Autodesk Fusion 360 part; units mm, degrees
sketch "Sketch1" plane through (0, 0, 0) normal (0, 0, 1) x (1, 0, 0)
  circle A0 centre (0, 0) radius 45.72 construction
  circle A1 centre (22.86, 39.5947) radius 4.4196
  line L0 (0, 0) -> (0, 63.5) construction
  line L1 (22.86, 39.5947) -> (0, 0) construction
  line L2 (0, 0) -> (69.088, 0) construction
  circle A2 centre (-22.86, 39.5947) radius 4.4196
  circle A3 centre (-45.72, 0) radius 4.4196
  circle A4 centre (-22.86, -39.5947) radius 4.4196
  circle A5 centre (22.86, -39.5947) radius 4.4196
  arc A6 (-14.8961, 45.9035) -> (-32.3056, 35.8522) centre (-22.86, 39.5947) ccw
  arc A7 (-47.2017, 10.0514) -> (-47.2017, -10.0514) centre (-45.72, 0) ccw
  arc A8 (-32.3056, -35.8522) -> (-14.8961, -45.9035) centre (-22.86, -39.5947) ccw
  line L3 (55.88, 55.88) -> (55.88, -43.18) construction
  arc A9 (22.2359, 30.9383) -> (41.7373, 32.3706) centre (31.1302, 43.3136) ccw
  arc A10 (45.7196, 0.1826) -> (46.0426, 0) centre (55.88, 17.78) ccw
  arc A11 (72.3846, 5.9267) -> (41.7373, 32.3706) centre (55.88, 17.78) ccw
  circle A12 centre (69.088, 48.26) radius 4.4196
  line L4 (-14.8961, 45.9035) -> (67.577, 58.307)
  line L5 (88.9, 25.4) -> (88.9, -25.4)
  line L6 (88.9, 25.4) -> (78.5547, 51.9489)
  circle A13 centre (79.248, 0) radius 4.4196
  arc A14 (22.2359, 30.9383) -> (22.2359, -30.9383) centre (0, 0) ccw
  arc A15 (0.7353, 48.2544) -> (0, 48.26) centre (0, 0) ccw
  arc A16 (78.5547, 51.9489) -> (67.577, 58.307) centre (69.088, 48.26) ccw
  line L7 (-14.8961, -45.9035) -> (67.577, -58.307)
  arc A17 (67.577, -58.307) -> (78.5547, -51.9489) centre (69.088, -48.26) ccw
  line L8 (88.9, -25.4) -> (78.5547, -51.9489)
  arc A18 (41.7373, -32.3706) -> (72.3846, -5.9267) centre (55.88, -17.78) ccw
  arc A19 (41.7373, -32.3706) -> (22.2359, -30.9383) centre (31.1302, -43.3136) ccw
  arc A20 (-32.3056, 35.8522) -> (-47.2017, 10.0514) centre (0, 0) ccw
  arc A21 (-47.2017, -10.0514) -> (-32.3056, -35.8522) centre (0, 0) ccw
  circle A22 centre (69.088, -48.26) radius 4.4196
  arc A23 (72.3846, 5.9267) -> (72.3846, -5.9267) centre (80.6369, 0) ccw
  dimension "d2" = 91.44
  dimension "d3" = 76.2
  dimension "d4" = 8.8392
  dimension "d5" = 30
  dimension "d7" = 240
  dimension "d13" = 55.88
  dimension "d14" = 40.64
  dimension "d15" = 17.78
  dimension "d16" = 30.48
  dimension "d17" = 8.8392
  dimension "d18" = 48.26
  dimension "d19" = 69.088
  dimension "d20" = 20.32
  dimension "d21" = 134.62
  dimension "d22" = 25.4
  dimension "d23" = 8.8392
  dimension "d24" = 79.248
  dimension "d28" = 20.32
extrude "Extrude1" add sketch "Sketch1" along normal mid plane 2.032
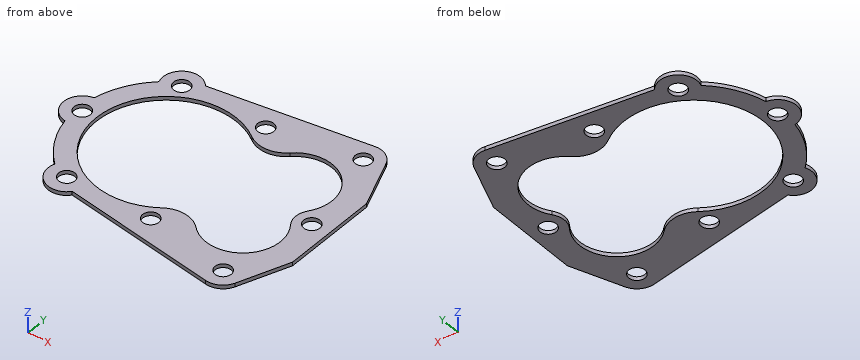
Model file for the job. Use its own axes, mm. Round coordinates to 2 decimals unless told otherwise and drop trailing zeros. Write each loop counter-clockwise with the first axis right and the second up, starting at its lowest first coordinate (ties: lowest second). Pieces come first, ordered by that corner, then holes. Notation, with made-up numbers: (-5, 72.5) - (16, 72.5) arc R22 cw to (16, 105.5) - close; hole circle Ø4 at (25.25, -16.5). An arc over 180 degrees is marked (long way). One line per item, written item: value.
(1) Cut at A-A, the plane y = 0. Give the cut face in (x, z).
Values follow:
outline: (-55.88, -1.02) - (-50.14, -1.02) - (-50.14, 1.02) - (-55.88, 1.02) - close; (-41.3, -1.02) - (-38.1, -1.02) - (-38.1, 1.02) - (-41.3, 1.02) - close; (70.48, -1.02) - (74.83, -1.02) - (74.83, 1.02) - (70.48, 1.02) - close; (83.67, -1.02) - (88.9, -1.02) - (88.9, 1.02) - (83.67, 1.02) - close
(2) Cut at C-C, the plane x = 12.5. Give the cut face in (y, z), plus the area to 3 significant figures.
Values follow:
outline: (-50.02, -1.02) - (-35.99, -1.02) - (-35.99, 1.02) - (-50.02, 1.02) - close; (35.99, -1.02) - (50.02, -1.02) - (50.02, 1.02) - (35.99, 1.02) - close
area: 57.0 mm²
(3) Cut at D-D, the plane y = 48.26. Give the cut face in (x, z), plus the area to 3 significant figures.
Values follow:
outline: (-28.16, -1.02) - (-17.56, -1.02) - (-17.56, 1.02) - (-28.16, 1.02) - close; (0.77, -1.02) - (64.67, -1.02) - (64.67, 1.02) - (0.77, 1.02) - close; (73.51, -1.02) - (79.99, -1.02) - (79.99, 1.02) - (73.51, 1.02) - close
area: 165 mm²
(4) Cut at B-B, the plane x = -22.86. Give the cut face in (y, z), plus the area to 3 significant figures.
Values follow:
outline: (-49.75, -1.02) - (-44.01, -1.02) - (-44.01, 1.02) - (-49.75, 1.02) - close; (-35.18, -1.02) - (-30.48, -1.02) - (-30.48, 1.02) - (-35.18, 1.02) - close; (30.48, -1.02) - (35.18, -1.02) - (35.18, 1.02) - (30.48, 1.02) - close; (44.01, -1.02) - (49.75, -1.02) - (49.75, 1.02) - (44.01, 1.02) - close
area: 42.4 mm²
(5) Drop flat-ended pins along their axis: P1, Ø14, axis at x = 22.86, y = 39.59, coming from the +Z side; P2, Ø1, axis at y = 3.5, z = -0.5, coming from the -X side; P3, Ø5.5, axis at x = -45.72, y = 0, coming from the -Z side; P4, Ø1, axis at y = 27, z = 0.5, coming from the +X side. Give the stop position or say it passes through.
Values follow:
P1: stops at z = 1.02
P2: stops at x = -55.43
P3: passes through
P4: stops at x = 88.47
(6) Wall check: probe 1 along Y at (x, z) = (-22.86, 0.1); probe 2 along Y at (x, z) = (22.86, 0.2); probe 3 along X at (y, z) = (-43.5, -0.5). Give the ranges that are in metal, low to high.
Values follow:
probe 1: y = -49.75 to -44.01, -35.18 to -30.48, 30.48 to 35.18, 44.01 to 49.75
probe 2: y = -51.58 to -44.01, -35.18 to -30.51, 30.51 to 35.18, 44.01 to 51.58
probe 3: x = -32.24 to -24.93, -20.79 to 20.79, 24.93 to 81.85
